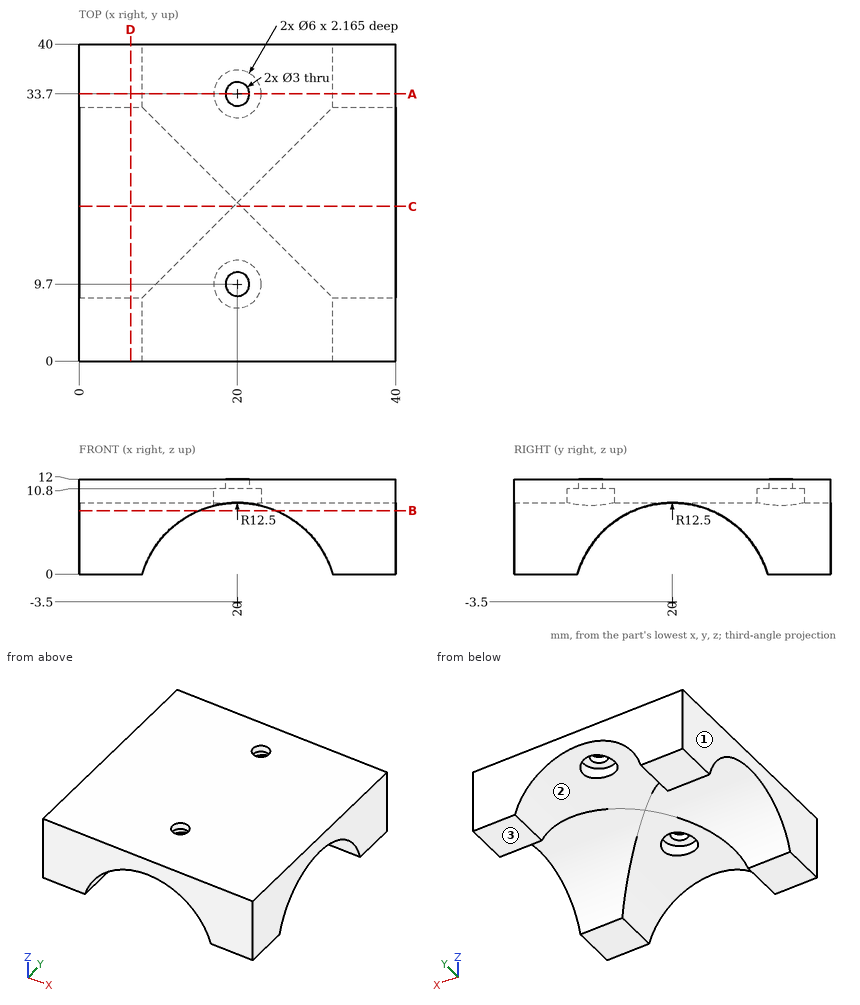
Design review of the part shown in the three views and the two pictorial views. Dimensions are in mm from the part's minimum x, y and z. Coordinates: 2 decimals unless noted, no trailing zeros. Order: outer loops, then holes, each group sorted by start corner. A loop starts at its lowest first (then second) coordinate and runs counter-clockwise, first axis right, second up.
Item 1: Take a section at D-D, the plane x = 6.5. Write out the cut boundary in (y, z), then the cut area to 3 significant figures.
Item 2: Take a section at C-C, the plane y = 19.5. Write out the cut boundary in (x, z), then the cut area to 3 significant figures.
Item 3: For pin 1 Ø8 at (x, y) = (20, 9.7) entering from -Z; pin 2 Ø3 at (x, y) = (19.5, 34) entering from -Z; pin 3 Ø10 at (x, y) = (10.5, 34.5) entering from -Z; pin 4 Ø6.5 at (x, y) = (20, 11) entering from -Z, all flat-tipped, find the tip position at first contact; note any pin that passes through.
Item 4: For line 1 (Y direction, x = 20, z = 10.25); line 2 (Y direction, x = 20, z = 11.3); line 3 (Y direction, x = 8, z = 1), list the stretches that pass through material, from the lowest coordinate up.
Item 5: Take a section at B-B, the plane z = 8. Write out the cut boundary in (x, y), then the cut area to 3 significant figures.
Item 6: Take a section at A-A, the plane y = 33.7. Write out the cut boundary in (x, z) (1 decimal), then the cut area to 3 significant figures.
Item 7: The part is to be moulded in two halves that separate along X. For the marked faces 1, 2 and 3, say which applies: pulls with the +X half, pulls with the -X half, needs draft (parallel to the pull), parting line crosses it, or undercut.
The answers:
1. outline: (0, 0) - (8, 0) arc R12.5 cw to (32, 0) - (40, 0) - (40, 12) - (0, 12) - close
1. area: 321 mm2
2. outline: (0, 8.99) - (19.5, 8.99) arc R12.5 cw to (20.5, 8.99) - (40, 8.99) - (40, 12) - (0, 12) - close
2. area: 120 mm2
3. pin 1: stops at z = 8.34
3. pin 2: stops at z = 10.8
3. pin 3: stops at z = 0
3. pin 4: stops at z = 8.57
4. line 1: y = 0 to 6.7, 12.7 to 30.7, 36.7 to 40
4. line 2: y = 0 to 8.2, 11.2 to 32.2, 35.2 to 40
4. line 3: y = 0 to 8.34, 31.66 to 40
5. outline: (0, 0) - (15.1, 0) - (15.1, 15.1) - (0, 15.1) - close; (0, 24.9) - (15.1, 24.9) - (15.1, 40) - (0, 40) - close; (24.9, 0) - (40, 0) - (40, 15.1) - (24.9, 15.1) - close; (24.9, 24.9) - (40, 24.9) - (40, 40) - (24.9, 40) - close
5. area: 912 mm2
6. outline: (0, 0) - (8, 0) arc R12.5 cw to (17, 8.6) - (17, 10.8) - (18.5, 10.8) - (18.5, 12) - (0, 12) - close; (21.5, 10.8) - (23, 10.8) - (23, 8.6) arc R12.5 cw to (32, 0) - (40, 0) - (40, 12) - (21.5, 12) - close
6. area: 306 mm2
7. face 1: pulls with the -X half
7. face 2: undercut
7. face 3: needs draft
